Autodesk Fusion 360 part; units mm, degrees
sketch "Sketch1" plane through (0, 0, 0) normal (0, 0, 1) x (1, 0, 0)
  line L0 (0, 0) -> (155, 0)
  line L1 (155, 0) -> (155, 21)
  line L2 (155, 21) -> (0, 21)
  line L3 (0, 21) -> (0, 0)
  dimension "d1" = 155
  dimension "d2" = 21
extrude "Extrude1" add sketch "Sketch1" along normal blind 85
sketch "Sketch2" plane through (0, 0, 85) normal (0, 0, 1) x (-1, 0, 0)
  line L0 (0, -21) -> (0, 0)
  line L1 (-155, 0) -> (-155, -21)
  line L2 (-155, -21) -> (0, -21)
shell "Shell1" thickness 5 removed faces 1 at (51.6667, 7, 85)
sketch "Sketch3" plane through (0, 0, 85) normal (0, 0, 1) x (-1, 0, 0)
sketch "Sketch4" plane through (0, 0, 85) normal (0, 0, 1) x (-1, 0, 0)
sketch "Sketch5" plane through (0, 0, 85) normal (0, 0, 1) x (-1, 0, 0)
sketch "Sketch6" plane through (0, 0, 85) normal (0, 0, 1) x (-1, 0, 0)
sketch "Sketch7" plane through (0, 0, 85) normal (0, 0, 1) x (-1, 0, 0)
sketch "Sketch8" plane through (0, 0, 85) normal (0, 0, 1) x (-1, 0, 0)
sketch "Sketch9" plane through (0, 0, 85) normal (0, 0, 1) x (-1, 0, 0)
sketch "Sketch10" plane through (0, 0, 85) normal (0, 0, 1) x (-1, 0, 0)
  line L0 (-140, 0) -> (-15, 0)
  line L1 (-15, 0) -> (-15, -21)
  line L2 (-15, -21) -> (-140, -21)
  line L3 (-140, -21) -> (-140, 0)
extrude "Extrude2" cut sketch "Sketch10" against normal blind 80
sketch "Sketch11" plane through (0, 0, 85) normal (0, 0, 1) x (-1, 0, 0)
  line L0 (-15, 0) -> (-15, -5)
  line L1 (-15, -5) -> (-5, -5)
  line L2 (-5, -5) -> (-5, -16)
  line L3 (-5, -16) -> (-15, -16)
  line L4 (-15, -16) -> (-15, -21)
  line L5 (-15, -21) -> (0, -21)
  line L6 (0, -21) -> (0, 0)
  line L7 (0, 0) -> (-15, 0)
  line L8 (-6, -13) -> (0, -13)
  line L9 (0, -8) -> (-6, -8)
  line L10 (-6, -13) -> (-155, -13)
  line L11 (-155, -13) -> (-155, -8)
  line L12 (-155, -8) -> (-6, -8)
  line L13 (0, -13) -> (0, -8)
extrude "Extrude3" cut sketch "Sketch11" against normal blind 80 contours L2 L6 L8 L9 L13 | L2 L8 L9 L10 L11 L12
sketch "Sketch12" plane through (0, 0, 85) normal (0, 0, 1) x (-1, 0, 0)
  line L0 (0, -13) -> (-5, -13)
  line L1 (-5, -13) -> (-5, -16)
  line L2 (-5, -16) -> (-15, -16)
  line L3 (-15, -16) -> (-15, -21)
  line L4 (-15, -21) -> (0, -21)
  line L5 (0, -21) -> (0, -13)
sketch "Sketch13" plane through (0, 0, 85) normal (0, 0, 1) x (-1, 0, 0)
  line L0 (0, -15) -> (-185, -15)
  line L1 (-185, -15) -> (-185, -6)
  line L2 (-185, -6) -> (0, -6)
  line L3 (0, -6) -> (0, -15)
  dimension "d10" = 185
extrude "Extrude4" cut sketch "Sketch13" against normal blind 80
sketch "Sketch14" plane through (15, 0, 0) normal (1, 0, 0) x (0, 1, 0)
  line L0 (5, 5) -> (5, 85)
  line L1 (5, 85) -> (0, 85)
  line L2 (0, 85) -> (0, 5)
  line L3 (0, 5) -> (5, 5)
  line L4 (0, 85) -> (5, 85)
  line L5 (5, 85) -> (5, 80)
  line L6 (5, 80) -> (0, 80)
  line L7 (0, 80) -> (0, 85)
  dimension "d13" = 5
  dimension "d14" = 5
extrude "Extrude5" add sketch "Sketch14" along normal blind 125 contours L0 L1 L2 L4 L5 L6 L7
sketch "Sketch15" plane through (15, 0, 0) normal (1, 0, 0) x (0, 1, 0)
  line L0 (16, 85) -> (16, 5)
  line L1 (16, 5) -> (21, 5)
  line L2 (21, 5) -> (21, 85)
  line L3 (21, 85) -> (16, 85)
  line L4 (21, 85) -> (16, 85)
  line L5 (16, 85) -> (16, 80)
  line L6 (16, 80) -> (21, 80)
  line L7 (21, 80) -> (21, 85)
  dimension "d17" = 5
extrude "Extrude6" add sketch "Sketch15" along normal blind 125 contours L0 L2 L3 L4 L5 L6 L7
sketch "Sketch16" plane through (0, 6, 0) normal (0, 1, 0) x (-1, 0, 0)
  line L0 (-5, 85) -> (-5, 5)
  line L1 (-5, 5) -> (0, 5)
  line L2 (0, 5) -> (0, 85)
  line L3 (0, 85) -> (-5, 85)
  line L4 (0, 85) -> (-5, 85)
  line L5 (-5, 85) -> (-5, 80)
  line L6 (-5, 80) -> (0, 80)
  line L7 (0, 80) -> (0, 85)
  dimension "d20" = 5
extrude "Extrude7" add sketch "Sketch16" along normal blind 10 contours L0 L2 L3 L4 L5 L6 L7
sketch "Sketch17" plane through (0, 6, 0) normal (0, 1, 0) x (-1, 0, 0)
  line L0 (-150, 5) -> (-150, 85)
  line L1 (-150, 85) -> (-155, 85)
  line L2 (-155, 85) -> (-155, 5)
  line L3 (-155, 5) -> (-150, 5)
  line L4 (-155, 85) -> (-150, 85)
  line L5 (-150, 85) -> (-150, 80)
  line L6 (-150, 80) -> (-155, 80)
  line L7 (-155, 80) -> (-155, 85)
extrude "Extrude8" add sketch "Sketch17" along normal blind 10 contours L0 L1 L2 L4 L5 L6 L7
Design review of the part built by this model. Coordinates are the model's own, in mm. A direction names the side the tool comes from. Round coordinates to 2 decimals unless told otherwise and drop trailing zeros. Loops run counter-clockwise (first coordinate to the right, second up) from the corner with the lowest first, then second, coordinate; pieces in that order, holes last. Notation, with made-up numbers: (48, 56) - (86, 56) arc R13 cw to (86, 78) - close; hole circle Ø6 at (10.25, 89). An arc over 180 degrees is marked (long way). One line per question, with ' | ' between items.
1. For faces 4 (the face through (152, 15, 43)), 5 (the face through (140, 19, 43)), 6 (the face through (79, 10, 5)), 7 (the face through (87.9, 5, 80.4)), list the 3-axis set-ups (+Z, -Z, +X, -X, +Y, -Y) from which the entire face can be reached by the end or side of a thin tool; tool diameter is ignored.
Results are:
face 4: +X, -X | face 5: +Y, -Y | face 6: none | face 7: +Z
2. We need section B-B, the plane x = 117.5. State the section outline as (y, z) points.
Results are:
outline: (0, 0) - (21, 0) - (21, 5) - (0, 5) - close; (0, 80) - (5, 80) - (5, 85) - (0, 85) - close; (16, 80) - (21, 80) - (21, 85) - (16, 85) - close
3. Clearance check with a flat-ended pin moving along its axis: P1, Ø9, axis at y = 9.5, z = 56, coming from the +X side. State where the tip first meets the part, or that it passes through.
Results are:
P1: stops at x = 155
4. We need section A-A, the plane z = 60.5. State the section outline as (x, y) points.
Results are:
outline: (0, 0) - (15, 0) - (15, 5) - (5, 5) - (5, 6) - (0, 6) - close; (0, 15) - (5, 15) - (5, 16) - (15, 16) - (15, 21) - (0, 21) - close; (140, 0) - (155, 0) - (155, 6) - (150, 6) - (150, 5) - (140, 5) - close; (140, 16) - (150, 16) - (150, 15) - (155, 15) - (155, 21) - (140, 21) - close
5. We need section C-C, the plane y = 9.5. State the section outline as (x, z) points.
Results are:
outline: (0, 0) - (155, 0) - (155, 5) - (0, 5) - close; (0, 80) - (5, 80) - (5, 85) - (0, 85) - close; (150, 80) - (155, 80) - (155, 85) - (150, 85) - close
6. For L1, parallel to X at y = 2, z = 42; L2, parallel to Z at x = 133, y = 1; L3, parallel to Y at x = 89.5, z = 81.5, list the stretches that pass through material, from the lowest coordinate up. Write a range as [from, to].
Results are:
L1: x = [0, 15], [140, 155] | L2: z = [0, 5], [80, 85] | L3: y = [0, 5], [16, 21]
7. Draft analysis for pull direction Y (two halves, no side actions). For faces 1 (the face through (71.4, 0, 80.5)), 2 (the face through (83, 16, 81)), 3 (the face through (140, 3, 43)), state which applies: released by +Y, released by -Y, zero draft, split by the parting line, or undercut.
Results are:
face 1: released by -Y | face 2: undercut | face 3: zero draft
